Here's how the part is built. I have some questions about the finished solid (model axes, mm). Round coordinates to 2 decimals unless told otherwise and drop trailing zeros. Order: outer loops, then holes, each group sorted by start corner. A loop starts at its lowest first (then second) coordinate and runs counter-clockwise, first axis right, second up. Notation, with made-up numbers: (54, 49) - (58, 49) arc R24 cw to (58, 81) - close; hole circle Ø8 at (55.25, 58). An arc over 180 degrees is marked (long way). Answer as a JSON object with one key per item and string values.
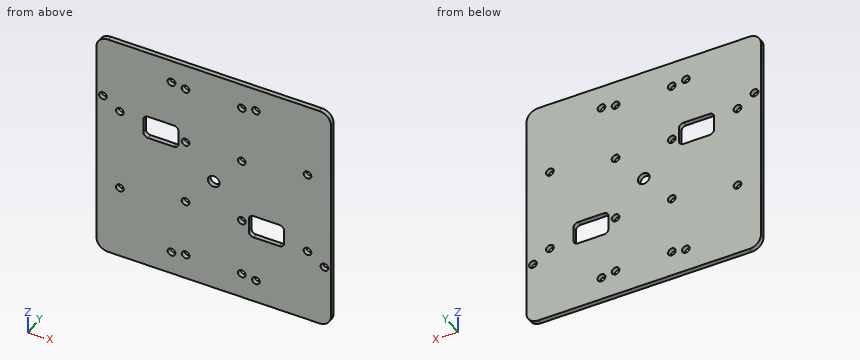
```python
from build123d import *

# Parameters (mm, degrees)
SKETCH_1_W               = 100
SKETCH_1_H               = 100
EXTRUDE_1_DEPTH          = 2
CUT_EXTRUDE_436_REACH    = 72.739
SKETCH_2_R               = 2.5
CUT_EXTRUDE_2_REACH      = 72.739
SKETCH_3_R               = 1.65
PATTERN_LINEAR_1_COUNT   = 2
PATTERN_LINEAR_1_PITCH   = 25
MIRROR_1_COPY_1_REACH    = 72.739
MIRROR_1_COPY_1_SKETCH_R = 1.65
CUT_EXTRUDE_3_REACH      = 72.739
SKETCH_5_R               = 1.65
PATTERN_CIRCULAR_1_COUNT = 2
CUT_EXTRUDE_4_REACH      = 72.739
SKETCH_6_R               = 1.65
PATTERN_CIRCULAR_2_COUNT = 2
PATTERN_CIRCULAR_2_ANGLE = 90
CUT_EXTRUDE_5_REACH      = 72.739
SKETCH_7_W               = 15
SKETCH_7_H               = 10
FILLET_1_R               = 2
FILLET_2_R               = 5


with BuildPart() as part:
    # Sketch 1 → Extrude 1 (new body)
    with BuildSketch(Plane(origin=(0, 0, 0), x_dir=(1, 0, 0), z_dir=(0, 1, 0))):
        Rectangle(SKETCH_1_W, SKETCH_1_H)
    extrude(amount=EXTRUDE_1_DEPTH)

    # Sketch 2 → Cut-Extrude 436 (cut, up to next)
    with BuildSketch(Plane(origin=(0, 2, 0), x_dir=(1, 0, 0), z_dir=(0, 1, 0)), mode=Mode.PRIVATE) as cut_extrude_436_sk1:
        with Locations(Location((0, 0, 0), (0, 0, 270))):
            Circle(SKETCH_2_R)
    cut_extrude_436_tool1 = extrude(cut_extrude_436_sk1.sketch, amount=-CUT_EXTRUDE_436_REACH, mode=Mode.PRIVATE) & part.part
    add(cut_extrude_436_tool1.solids().sort_by_distance((0, 2, 0))[0], mode=Mode.SUBTRACT)

    # Sketch 3 → Cut-Extrude 2 (cut, up to next)
    with BuildSketch(Plane(origin=(0, 2, 0), x_dir=(1, 0, 0), z_dir=(0, 1, 0)), mode=Mode.PRIVATE) as cut_extrude_2_sk1:
        with Locations(Location((-12, 39, 0), (0, 0, 270))):
            Circle(SKETCH_3_R)
    cut_extrude_2_tool1 = extrude(cut_extrude_2_sk1.sketch, amount=-CUT_EXTRUDE_2_REACH, mode=Mode.PRIVATE) & part.part
    # Sketch 3 → Cut-Extrude 2 (cut, up to next)
    with BuildSketch(Plane(origin=(0, 2, 0), x_dir=(1, 0, 0), z_dir=(0, 1, 0)), mode=Mode.PRIVATE) as cut_extrude_2_sk2:
        with Locations(Location((12, 39, 0), (0, 0, 270))):
            Circle(SKETCH_3_R)
    cut_extrude_2_tool2 = extrude(cut_extrude_2_sk2.sketch, amount=-CUT_EXTRUDE_2_REACH, mode=Mode.PRIVATE) & part.part
    cut_extrude_2_1 = cut_extrude_2_tool1.solids().sort_by_distance((-12, 2, -39))[0]
    add(cut_extrude_2_1, mode=Mode.SUBTRACT)
    cut_extrude_2_2 = cut_extrude_2_tool2.solids().sort_by_distance((12, 2, -39))[0]
    add(cut_extrude_2_2, mode=Mode.SUBTRACT)
    cut_extrude_2 = cut_extrude_2_1 + cut_extrude_2_2  # Cut-Extrude 2 as one shape, for the pattern or mirror that repeats it

    # Pattern Linear 1: Cut-Extrude 2 ×2
    with Locations(*[(0, 0, i * PATTERN_LINEAR_1_PITCH) for i in range(1, PATTERN_LINEAR_1_COUNT)]):
        add(cut_extrude_2, mode=Mode.SUBTRACT)

    # Mirror 1: Cut-Extrude 2 across plane
    add(cut_extrude_2.mirror(Plane.XY), mode=Mode.SUBTRACT)

    # Mirror 1 copy 1 sketch → Mirror 1 copy 1 (cut, up to next)
    with BuildSketch(Plane(origin=(0, 2, -25), x_dir=(1, 0, 0), z_dir=(0, 1, 0)), mode=Mode.PRIVATE) as mirror_1_copy_1_sk1:
        with Locations((-12, -39)):
            Circle(MIRROR_1_COPY_1_SKETCH_R)
    mirror_1_copy_1_tool1 = extrude(mirror_1_copy_1_sk1.sketch, amount=-MIRROR_1_COPY_1_REACH, mode=Mode.PRIVATE) & part.part
    # Mirror 1 copy 1 sketch → Mirror 1 copy 1 (cut, up to next)
    with BuildSketch(Plane(origin=(0, 2, -25), x_dir=(1, 0, 0), z_dir=(0, 1, 0)), mode=Mode.PRIVATE) as mirror_1_copy_1_sk2:
        with Locations((12, -39)):
            Circle(MIRROR_1_COPY_1_SKETCH_R)
    mirror_1_copy_1_tool2 = extrude(mirror_1_copy_1_sk2.sketch, amount=-MIRROR_1_COPY_1_REACH, mode=Mode.PRIVATE) & part.part
    add(mirror_1_copy_1_tool1.solids().sort_by_distance((-12, 2, 14))[0], mode=Mode.SUBTRACT)
    add(mirror_1_copy_1_tool2.solids().sort_by_distance((12, 2, 14))[0], mode=Mode.SUBTRACT)

    # Sketch 5 → Cut-Extrude 3 (cut, up to next)
    with BuildSketch(Plane(origin=(0, 2, 0), x_dir=(1, 0, 0), z_dir=(0, 1, 0)), mode=Mode.PRIVATE) as cut_extrude_3_sk1:
        with Locations(Location((47.25, 22.75, 0), (0, 0, 270))):
            Circle(SKETCH_5_R)
    cut_extrude_3_tool1 = extrude(cut_extrude_3_sk1.sketch, amount=-CUT_EXTRUDE_3_REACH, mode=Mode.PRIVATE) & part.part
    cut_extrude_3 = cut_extrude_3_tool1.solids().sort_by_distance((47.25, 2, -22.75))[0]
    add(cut_extrude_3, mode=Mode.SUBTRACT)

    # Pattern Circular 1: Cut-Extrude 3 ×2 about axis
    pattern_circular_1_axis = Axis((0, 0, 0), (0, 1, 0))
    for i in range(1, PATTERN_CIRCULAR_1_COUNT):
        add(cut_extrude_3.rotate(pattern_circular_1_axis, i * 360 / PATTERN_CIRCULAR_1_COUNT), mode=Mode.SUBTRACT)

    # Sketch 6 → Cut-Extrude 4 (cut, up to next)
    with BuildSketch(Plane(origin=(0, 2, 0), x_dir=(1, 0, 0), z_dir=(0, 1, 0)), mode=Mode.PRIVATE) as cut_extrude_4_sk1:
        with Locations(Location((-40, 18, 0), (0, 0, 270))):
            Circle(SKETCH_6_R)
    cut_extrude_4_tool1 = extrude(cut_extrude_4_sk1.sketch, amount=-CUT_EXTRUDE_4_REACH, mode=Mode.PRIVATE) & part.part
    # Sketch 6 → Cut-Extrude 4 (cut, up to next)
    with BuildSketch(Plane(origin=(0, 2, 0), x_dir=(1, 0, 0), z_dir=(0, 1, 0)), mode=Mode.PRIVATE) as cut_extrude_4_sk2:
        with Locations(Location((-40, -18, 0), (0, 0, 270))):
            Circle(SKETCH_6_R)
    cut_extrude_4_tool2 = extrude(cut_extrude_4_sk2.sketch, amount=-CUT_EXTRUDE_4_REACH, mode=Mode.PRIVATE) & part.part
    # Sketch 6 → Cut-Extrude 4 (cut, up to next)
    with BuildSketch(Plane(origin=(0, 2, 0), x_dir=(1, 0, 0), z_dir=(0, 1, 0)), mode=Mode.PRIVATE) as cut_extrude_4_sk3:
        with Locations(Location((40, -18, 0), (0, 0, 270))):
            Circle(SKETCH_6_R)
    cut_extrude_4_tool3 = extrude(cut_extrude_4_sk3.sketch, amount=-CUT_EXTRUDE_4_REACH, mode=Mode.PRIVATE) & part.part
    # Sketch 6 → Cut-Extrude 4 (cut, up to next)
    with BuildSketch(Plane(origin=(0, 2, 0), x_dir=(1, 0, 0), z_dir=(0, 1, 0)), mode=Mode.PRIVATE) as cut_extrude_4_sk4:
        with Locations(Location((40, 18, 0), (0, 0, 270))):
            Circle(SKETCH_6_R)
    cut_extrude_4_tool4 = extrude(cut_extrude_4_sk4.sketch, amount=-CUT_EXTRUDE_4_REACH, mode=Mode.PRIVATE) & part.part
    cut_extrude_4_1 = cut_extrude_4_tool1.solids().sort_by_distance((-40, 2, -18))[0]
    add(cut_extrude_4_1, mode=Mode.SUBTRACT)
    cut_extrude_4_2 = cut_extrude_4_tool2.solids().sort_by_distance((-40, 2, 18))[0]
    add(cut_extrude_4_2, mode=Mode.SUBTRACT)
    cut_extrude_4_3 = cut_extrude_4_tool3.solids().sort_by_distance((40, 2, 18))[0]
    add(cut_extrude_4_3, mode=Mode.SUBTRACT)
    cut_extrude_4_4 = cut_extrude_4_tool4.solids().sort_by_distance((40, 2, -18))[0]
    add(cut_extrude_4_4, mode=Mode.SUBTRACT)
    cut_extrude_4 = cut_extrude_4_1 + cut_extrude_4_2 + cut_extrude_4_3 + cut_extrude_4_4  # Cut-Extrude 4 as one shape, for the pattern or mirror that repeats it

    # Pattern Circular 2: Cut-Extrude 4 ×2 about axis
    pattern_circular_2_axis = Axis((0, 0, 0), (0, -1, 0))
    for i in range(1, PATTERN_CIRCULAR_2_COUNT):
        add(cut_extrude_4.rotate(pattern_circular_2_axis, i * PATTERN_CIRCULAR_2_ANGLE / (PATTERN_CIRCULAR_2_COUNT - 1)), mode=Mode.SUBTRACT)

    # Sketch 7 → Cut-Extrude 5 (cut, up to next)
    with BuildSketch(Plane(origin=(0, 2, 0), x_dir=(1, 0, 0), z_dir=(0, 1, 0)), mode=Mode.PRIVATE) as cut_extrude_5_sk1:
        with Locations((-22.5, -15)):
            Rectangle(SKETCH_7_W, SKETCH_7_H)
    cut_extrude_5_tool1 = extrude(cut_extrude_5_sk1.sketch, amount=-CUT_EXTRUDE_5_REACH, mode=Mode.PRIVATE) & part.part
    # Sketch 7 → Cut-Extrude 5 (cut, up to next)
    with BuildSketch(Plane(origin=(0, 2, 0), x_dir=(1, 0, 0), z_dir=(0, 1, 0)), mode=Mode.PRIVATE) as cut_extrude_5_sk2:
        with Locations((22.5, 15)):
            Rectangle(SKETCH_7_W, SKETCH_7_H)
    cut_extrude_5_tool2 = extrude(cut_extrude_5_sk2.sketch, amount=-CUT_EXTRUDE_5_REACH, mode=Mode.PRIVATE) & part.part
    add(cut_extrude_5_tool1.solids().sort_by_distance((-22.5, 2, 15))[0], mode=Mode.SUBTRACT)
    add(cut_extrude_5_tool2.solids().sort_by_distance((22.5, 2, -15))[0], mode=Mode.SUBTRACT)

    # Fillet 1
    fillet_1_edges = [part.edges().sort_by_distance(p)[0] for p in [
        (15, 1, -10),
        (15, 1, -20),
        (30, 1, -20),
        (30, 1, -10),
        (-15, 1, 10),
        (-15, 1, 20),
        (-30, 1, 20),
        (-30, 1, 10),
    ]]
    fillet(fillet_1_edges, radius=FILLET_1_R)

    # Fillet 2
    fillet_2_edges = [part.edges().sort_by_distance(p)[0] for p in [
        (50, 1, 50),
        (-50, 1, 50),
        (-50, 1, -50),
        (50, 1, -50),
    ]]
    fillet(fillet_2_edges, radius=FILLET_2_R)


solid = part.part
```
1. Imagine slicing it at C-C (x = -26.5). List the corners of the cut face in (y, z) for me, plus the area to 3 significant figures.
Responses:
{"outline": "(0, -50) - (2, -50) - (2, 10) - (0, 10) - close; (0, 20) - (2, 20) - (2, 50) - (0, 50) - close", "area": "180 mm2"}
2. Imagine slicing it at A-A (x = 12). List the corners of the cut face in (y, z) for me, plus the area to 3 significant figures.
Responses:
{"outline": "(0, -50) - (2, -50) - (2, -40.65) - (0, -40.65) - close; (0, -37.35) - (2, -37.35) - (2, -15.65) - (0, -15.65) - close; (0, -12.35) - (2, -12.35) - (2, 12.35) - (0, 12.35) - close; (0, 15.65) - (2, 15.65) - (2, 37.35) - (0, 37.35) - close; (0, 40.65) - (2, 40.65) - (2, 50) - (0, 50) - close", "area": "174 mm2"}
3. If I drill on L1, parallel to X at y = 1.1, z = 18; L2, parallel to Z at x = -23, y = 0.9; L3, parallel to Z at x = 11, y = 1.05, over which ranges is the centre line in solid material (lowest first)? Write a range as [from, to].
Responses:
{"L1": "[-50, -41.65], [-38.35, -30], [-15, 38.35], [41.65, 50]", "L2": "[-50, 10], [20, 50]", "L3": "[-50, -40.31], [-37.69, -15.31], [-12.69, 12.69], [15.31, 37.69], [40.31, 50]"}
4. Imagine slicing it at D-D (x = 40). List the corners of the cut face in (y, z) for me.
Responses:
{"outline": "(0, -50) - (2, -50) - (2, -19.65) - (0, -19.65) - close; (0, -16.35) - (2, -16.35) - (2, 16.35) - (0, 16.35) - close; (0, 19.65) - (2, 19.65) - (2, 50) - (0, 50) - close"}
5. Imagine slicing it at B-B (z = 14). List the corners of the cut face in (x, y) for me, plus the area to 3 significant figures.
Responses:
{"outline": "(-50, 0) - (-30, 0) - (-30, 2) - (-50, 2) - close; (-15, 0) - (-13.65, 0) - (-13.65, 2) - (-15, 2) - close; (-10.35, 0) - (10.35, 0) - (10.35, 2) - (-10.35, 2) - close; (13.65, 0) - (50, 0) - (50, 2) - (13.65, 2) - close", "area": "157 mm2"}
